Build history of the part. All positions in model axes, mm. Face numbers are marked on the shaded views. A direction names the side the tool comes from. Round coordinates to 2 decimals unless told otherwise and drop trailing zeros. Write each loop counter-clockwise with the first axis right and the second up, starting at its lowest first coordinate (ties: lowest second). Pieces come first, ordered by that corner, then holes. Notation, with made-up numbers: (53, -24.75) -> (58, -24.75) arc R18 cw to (58, -18.75) -> close; hole circle Ø3 at (63.5, 64.5). An arc over 180 degrees is marked (long way). One line per question, with ' | ' between items.
from build123d import *

# Parameters (mm, degrees)
SKETCH1_R           = 5
BOSS_EXTRUDE1_DEPTH = 0.5
SKETCH2_R           = 3.9
BOSS_EXTRUDE2_DEPTH = 4.5
SKETCH4_R           = 1
CUT_EXTRUDE1_DEPTH  = 4.5
CUT_EXTRUDE2_REACH  = 10.958
SKETCH5_R           = 0.9
CHAMFER1_SIZE       = 0.2


with BuildPart() as part:
    # Sketch1 → Boss-Extrude1 (new, symmetric)
    with BuildSketch(Plane(origin=(0, 0, 0), x_dir=(1, 0, 0), z_dir=(0, 1, 0))):
        with Locations(Location((0, 0, 0), (0, 0, 270))):
            Circle(SKETCH1_R)
    extrude(amount=BOSS_EXTRUDE1_DEPTH, both=True)

    # Sketch2 → Boss-Extrude2 (add)
    with BuildSketch(Plane(origin=(0, -0.5, 0), x_dir=(-1, 0, 0), z_dir=(0, -1, 0))):
        with Locations(Location((0, 0, 0), (0, 0, 270))):
            Circle(SKETCH2_R)
    extrude(amount=BOSS_EXTRUDE2_DEPTH)

    # Sketch4 → Cut-Extrude1 (cut)
    with BuildSketch(Plane(origin=(0, -5, 0), x_dir=(-1, 0, 0), z_dir=(0, -1, 0))):
        with Locations(Location((0, 0, 0), (0, 0, 90))):
            Circle(SKETCH4_R)
    extrude(amount=-CUT_EXTRUDE1_DEPTH, mode=Mode.SUBTRACT)

    # Sketch5 → Cut-Extrude2 (cut, up to next)
    with BuildSketch(Plane(origin=(0, 0.5, 0), x_dir=(1, 0, 0), z_dir=(0, 1, 0)), mode=Mode.PRIVATE) as cut_extrude2_sk1:
        with Locations(Location((0, 0, 0), (0, 0, 270))):
            Circle(SKETCH5_R)
    cut_extrude2_tool1 = extrude(cut_extrude2_sk1.sketch, amount=-CUT_EXTRUDE2_REACH, mode=Mode.PRIVATE) & part.part
    add(cut_extrude2_tool1.solids().sort_by_distance((0, 0.5, 0))[0], mode=Mode.SUBTRACT)

    # Chamfer1
    chamfer1_edges = [part.edges().sort_by_distance(p)[0] for p in [
        (0, -5, 1),
    ]]
    chamfer(chamfer1_edges, length=CHAMFER1_SIZE)


solid = part.part
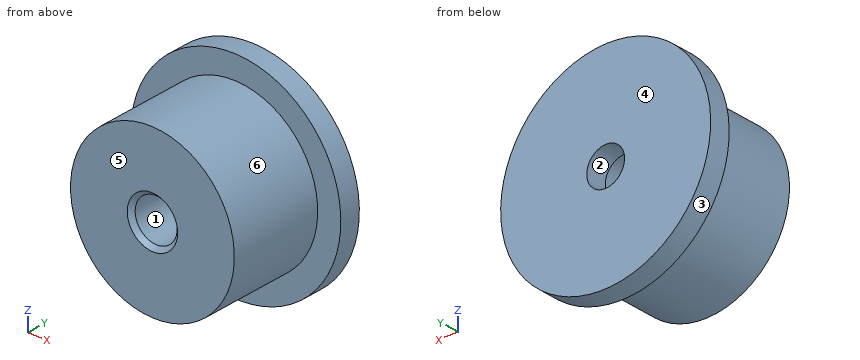
(1) 3-axis set-ups, long thin cutter, end or side, ignore diameter. For the marked faces 5 and 6: which of +Z, -Z, +X, -X, +Y, -Y reach the whole face in a straight line?
Calculated:
face 5: +Z, -Z, +X, -X, -Y | face 6: -Y
(2) Slice it at C-C (y = -0.35). Write the cut outline in (x, z).
Calculated:
outline: circle Ø10 at (0, 0); hole circle Ø1.8 at (0, 0)
(3) Slice it at B-B (z = 0). Write the cut outline in (x, y).
Calculated:
outline: (-5, -0.5) -> (-3.9, -0.5) -> (-3.9, -5) -> (-1.2, -5) -> (-1, -4.8) -> (-1, -0.5) -> (-0.9, -0.5) -> (-0.9, 0.5) -> (-5, 0.5) -> close; (0.9, -0.5) -> (1, -0.5) -> (1, -4.8) -> (1.2, -5) -> (3.9, -5) -> (3.9, -0.5) -> (5, -0.5) -> (5, 0.5) -> (0.9, 0.5) -> close
(4) Wall check: line 1 (X direction, y = -1.5, z = 0); line 2 (X direction, y = -0.15, z = 0); line 3 (Y direction, x = 0.5, z = 4.75). Give the ranges that are in metal, low to high. Write a range as from..to.
Calculated:
line 1: -3.9..-1, 1..3.9 | line 2: -5..-0.9, 0.9..5 | line 3: -0.5..0.5
(5) Slice it at D-D (z = -3.75). Write the cut outline in (x, y), then the cut area to 3 significant figures.
Calculated:
outline: (-3.31, -0.5) -> (-1.07, -0.5) -> (-1.07, -5) -> (1.07, -5) -> (1.07, -0.5) -> (3.31, -0.5) -> (3.31, 0.5) -> (-3.31, 0.5) -> close | area: 16.3 mm2
(6) Drop flat-ended pins along their axis: pin 1 (1.5 mm diameter, centred on x = -3.5, y = -1, fed in from -Z); pin 2 (3 mm diameter, centred on y = -0.5, z = 3.5, fed in from +X); pin 3 (2 mm diameter, centred on y = 0, z = -3.5, fed in from +X). Give the stop position or say it passes through.
Calculated:
pin 1: z = -4.04 | pin 2: x = 4.58 | pin 3: x = 4.33
(7) Mould opens along Z. For the marked faces 1, 2, 3 and 4 say: pulls with the +Z half, pulls with the -Z half, needs draft (parallel to the pull), parting line crosses it, or undercut.
Calculated:
face 1: undercut | face 2: undercut | face 3: parting line crosses it | face 4: needs draft
(8) Slice it at A-A (x = 0). Write the cut outline in (y, z).
Calculated:
outline: (-5, -3.9) -> (-0.5, -3.9) -> (-0.5, -5) -> (0.5, -5) -> (0.5, -0.9) -> (-0.5, -0.9) -> (-0.5, -1) -> (-4.8, -1) -> (-5, -1.2) -> close; (-5, 1.2) -> (-4.8, 1) -> (-0.5, 1) -> (-0.5, 0.9) -> (0.5, 0.9) -> (0.5, 5) -> (-0.5, 5) -> (-0.5, 3.9) -> (-5, 3.9) -> close
